Can you work these out from the drawing? Everything is in mm from the part's minimum corner. Give positions to 0.01 mm unless a question says otherwise; leave off trailing zeros. Write each loop counter-clockwise with the first axis right and the second up, starting at its lowest first coordinate (ties: lowest second). Pieces come first, ordered by that corner, then holes. Notation, with made-up numbers: (-34.5, 42) -> (4.5, 42) arc R10 cw to (4.5, 50) -> close; hole circle Ø9 at (-2, 56.5). An arc over 180 degrees is marked (long way). Return JSON: item names as keys, results as strings.
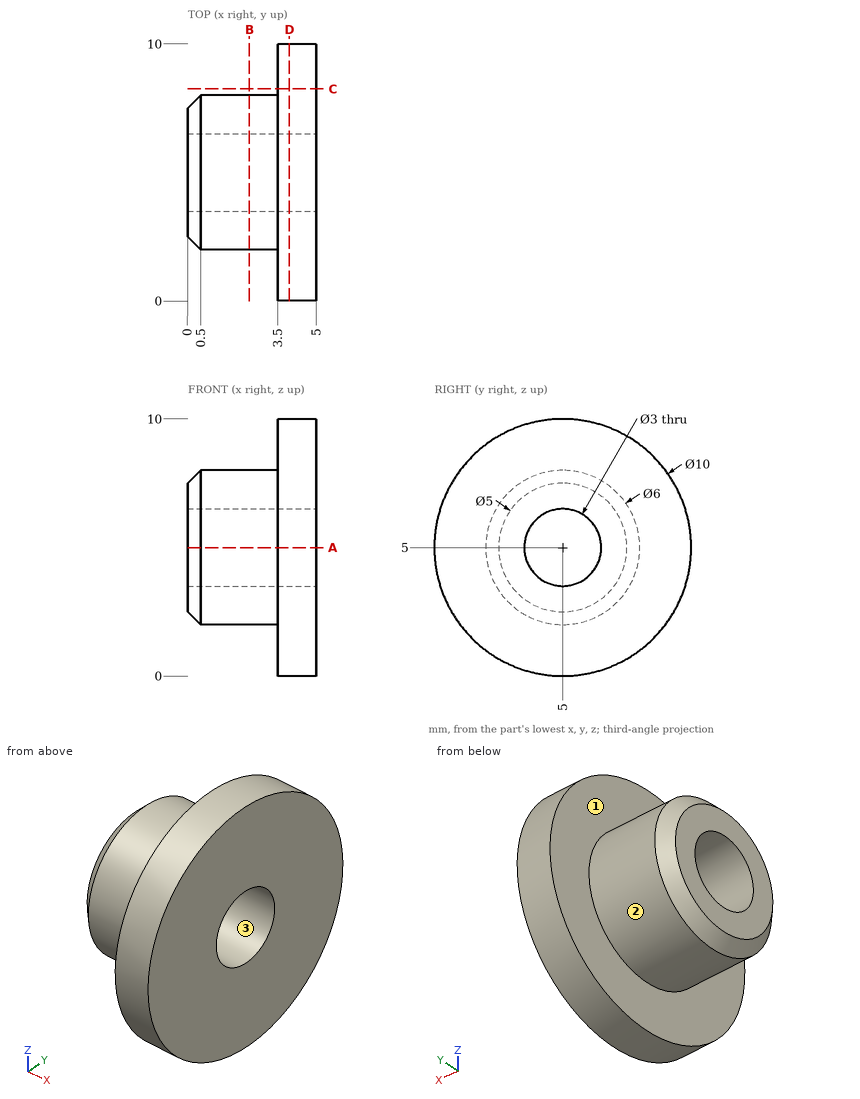
1. Suppose I cut it at D-D, the plane x = 3.95. List the corners of the cut face in (y, z) for me, and give its area (3 significant figures).
Taken from the geometry:
{"outline": "circle Ø10 at (5, 5); hole circle Ø3 at (5, 5)", "area": "71.5 mm²"}
2. If I drill on line 1 (Y direction, x = 1.75, z = 5); line 2 (Y direction, x = 3.7, z = 5); line 3 (X direction, y = 2, z = 7.25), over which ranges is the centre line in solid material (lowest first)? Write a range as [from, to].
Taken from the geometry:
{"line 1": "y = [2, 3.5], [6.5, 8]", "line 2": "y = [0, 3.5], [6.5, 10]", "line 3": "x = [3.5, 5]"}
3. If we mould it in two halves opening along Z, with no side actions, what happens to the marked faces 1, 2 and 3? For each: released by +Z, released by -Z, zero draft, split by the parting line, or undercut.
Taken from the geometry:
{"face 1": "zero draft", "face 2": "split by the parting line", "face 3": "undercut"}
4. Suppose I cut it at B-B, the plane x = 2.4. List the corners of the cut face in (y, z) for me, and give its area (3 significant figures).
Taken from the geometry:
{"outline": "circle Ø6 at (5, 5); hole circle Ø3 at (5, 5)", "area": "21.2 mm²"}
5. Suppose I cut it at A-A, the plane z = 5. List the corners of the cut face in (x, y) for me.
Taken from the geometry:
{"outline": "(0, 2.5) -> (0.5, 2) -> (3.5, 2) -> (3.5, 0) -> (5, 0) -> (5, 3.5) -> (0, 3.5) -> close; (0, 6.5) -> (5, 6.5) -> (5, 10) -> (3.5, 10) -> (3.5, 8) -> (0.5, 8) -> (0, 7.5) -> close"}
6. Suppose I cut it at C-C, the plane y = 8.25. List the corners of the cut face in (x, z) for me.
Taken from the geometry:
{"outline": "(3.5, 1.2) -> (5, 1.2) -> (5, 8.8) -> (3.5, 8.8) -> close"}
7. For pin 1 Ø1 at (x, y) = (2.5, 5.5) entering from -Z; pin 2 Ø2.5 at (y, z) = (5, 5) entering from +X; pin 3 Ø1 at (y, z) = (8, 9) entering from -X; pin 4 Ø3 at (y, z) = (4, 8) entering from -X, each with a flat end and sliding along its axis, tell me the tip position at first contact or that it passes through.
Taken from the geometry:
{"pin 1": "stops at z = 2", "pin 2": "passes through", "pin 3": "stops at x = 3.5", "pin 4": "stops at x = 0"}
